Autodesk Fusion 360 part; units mm, degrees
sketch "スケッチ1" plane through (0, 0, 0) normal (0, 0, 1) x (1, 0, 0)
  line L0 (-3.5, 163) -> (-86.5, 163)
  line L1 (-86.5, 163) -> (-86.5, -163)
  line L2 (-86.5, -163) -> (-3.5, -163)
  line L3 (86.5, -5) -> (86.5, 155)
  line L4 (82.2546, 155) -> (-86.5, -163) construction
  line L5 (-86.5, 163) -> (46.1223, -86.9125) construction
  line L6 (-3.5, 163) -> (-3.5, 155)
  line L7 (-3.5, 155) -> (86.5, 155)
  line L8 (-86.5, -163) -> (-3.5, -163) construction
  line L9 (-3.5, -163) -> (86.5, -25)
  line L10 (86.5, -25) -> (-3.5, -25)
  line L11 (-3.5, -25) -> (-3.5, -5)
  line L12 (-3.5, -5) -> (86.5, -5)
  dimension "d2" = 326
  dimension "d5" = 83
  dimension "d7" = 90
  dimension "d8" = 20
extrude "押し出し1" add sketch "スケッチ1" along normal blind 6
chamfer "面取り1" distance 30 angle 45 2 edges at (-86.5, -163, 3) (-86.5, 163, 3)
sketch "スケッチ2" plane through (0, 0, 6) normal (0, 0, 1) x (-1, 0, 0)
  line L0 (56.5, -163) -> (86.5, -133)
  line L1 (86.5, -133) -> (86.5, 133)
  line L2 (86.5, 133) -> (56.5, 163)
  line L3 (56.5, 163) -> (3.5, 163)
  line L4 (3.5, 163) -> (-86.5, 25)
  line L5 (-86.5, 25) -> (3.5, 25)
  line L6 (3.5, 25) -> (3.5, 5)
  line L7 (3.5, 5) -> (-86.5, 5)
  line L8 (-86.5, 5) -> (-86.5, -155)
  line L9 (-86.5, -155) -> (3.5, -155)
  line L10 (3.5, -155) -> (3.5, -163)
  line L11 (3.5, -163) -> (56.5, -163)
  line L12 (-86.5, -155) -> (-46.5, -155) construction
  line L13 (-46.5, -155) -> (-46.5, -105) construction
  line L14 (-46.5, -105) -> (-86.5, -105) construction
  line L15 (-86.5, -105) -> (-86.5, -155) construction
  line L16 (-46.5, -105) -> (-46.5, -45) construction
  point P0 (-46.5, -105)
  point P1 (-46.5, -45)
  dimension "d12" = 40
  dimension "d13" = 50
  dimension "d14" = 60
hole "穴1" at (46.5, 105, 6) at (46.5, 45, 6) direction (0, 0, -1) diameter 18 end through all
equation "d5 = 30 mm + 53 mm"
The listing builds one solid part. Answer for the finished solid, in the listing's coordinates (mm). A direction names the side the tool comes from. Give positions to 0.01 mm unless a question says otherwise; leave off trailing zeros. Write each loop counter-clockwise with the first axis right and the second up, starting at its lowest first coordinate (ties: lowest second). Pieces come first, ordered by that corner, then holes. Notation, with made-up numbers: (87.5, -20.75) -> (104.5, -20.75) arc R30 cw to (104.5, 18.25) -> close; hole circle Ø3 at (81.5, 42.5). An arc over 180 degrees is marked (long way). Use one line per item in the form item = value.
1) For a pull along Y with two mould halves and no side action, classify faces 4 (the flat face through (41, 155, 3)), 5 (the flat face through (-1, 2, 0)), 6 (the flat face through (42, -25, 3)), 7 (the flat face through (-71.7, -147.8, 3)) as +Y half, -Y half, draft (parallel to the pull), parting line (faces both ways), or undercut.
Result:
face_4 = +Y half
face_5 = draft
face_6 = undercut
face_7 = -Y half
2) Section A-A on y = 105 is taken. Write down the section's boundary in (x, z), plus the area to 3 significant figures.
Result:
outline = (-86.5, 0) -> (37.5, 0) -> (37.5, 6) -> (-86.5, 6) -> close; (55.5, 0) -> (86.5, 0) -> (86.5, 6) -> (55.5, 6) -> close
area = 930 mm²
3) Section C-C on x = 46.5 is taken. Write down the section's boundary in (y, z).
Result:
outline = (-86.33, 0) -> (-25, 0) -> (-25, 6) -> (-86.33, 6) -> close; (-5, 0) -> (36, 0) -> (36, 6) -> (-5, 6) -> close; (54, 0) -> (96, 0) -> (96, 6) -> (54, 6) -> close; (114, 0) -> (155, 0) -> (155, 6) -> (114, 6) -> close
4) Each of these flat-tipped pins is pushed along its axis until it touches: P1, Ø1.5, axis at x = 39.5, z = 4.5, coming from the +Y side; P2, Ø1.5, axis at y = -10.5, z = 3.5, coming from the +X side; P3, Ø3, axis at x = 58, z = 3.5, coming from the -Y side. Where does it stop, or does it pass through?
Result:
P1 = 155
P2 = -3.5
P3 = -71
5) A tool of negligible diameter and unlimited length cuts with its end or side. For faces 1 (the flat face through (-3.5, -15, 3)), 2 (the flat face through (-30, 163, 3)), 3 (the flat face through (-3.5, 159, 3)), from which of +Z, -Z, +X, -X, +Y, -Y can it reach the whole face along a straight path? Write none if from no direction.
Result:
face_1 = +Z, -Z, +X
face_2 = +Z, -Z, +X, -X, +Y
face_3 = +Z, -Z, +X, +Y
6) Straight lines are drawn through the part: probe 1 along Y at (x, z) = (66, 4.85); probe 2 along X at (y, z) = (105, 4.1); probe 3 along Y at (x, z) = (79, 2.5). For each, find the intervals that lie inside material, in ascending order.
Result:
probe_1 = -56.43 to -25, -5 to 155
probe_2 = -86.5 to 37.5, 55.5 to 86.5
probe_3 = -36.5 to -25, -5 to 155
7) Section B-B on z = 3.3 is taken. Write down the section's boundary in (x, y).
Result:
outline = (-86.5, -133) -> (-56.5, -163) -> (-3.5, -163) -> (86.5, -25) -> (-3.5, -25) -> (-3.5, -5) -> (86.5, -5) -> (86.5, 155) -> (-3.5, 155) -> (-3.5, 163) -> (-56.5, 163) -> (-86.5, 133) -> close; hole circle Ø18 at (46.5, 45); hole circle Ø18 at (46.5, 105)
8) Section D-D on y = -140 is taken. Write down the section's boundary in (x, z).
Result:
outline = (-79.5, 0) -> (11.5, 0) -> (11.5, 6) -> (-79.5, 6) -> close
